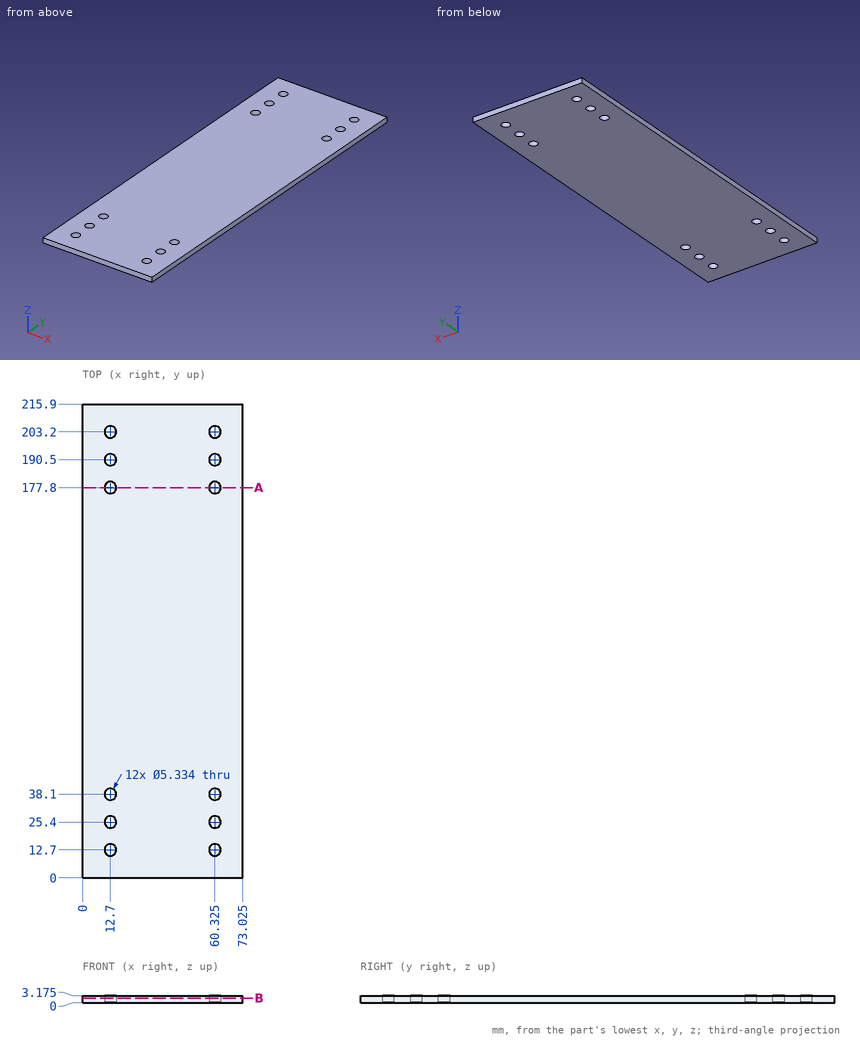
Part print with two shaded views. Sizes in mm from the minimum x, y, z corner. Coordinates: 2 decimals unless noted, no trailing zeros. Write each loop counter-clockwise with the first axis right and the second up, starting at its lowest first coordinate (ties: lowest second). Pieces come first, ordered by that corner, then holes.
1. Drill centre line: probe 1 along X at (y, z) = (177.8, 1.35) (3 decimals). Where is it in solid material? Low to high.
Answer block:
probe 1: x = 0 to 10.033, 15.367 to 57.658, 62.992 to 73.025
2. Drop a flat-ended pin along its axis: pin 1 (4.5 mm diameter, centred on x = 60.325, y = 25.4, fed in from +Z). Give the stop position or say it passes through.
Answer block:
pin 1: passes through
3. Band-saw the part on A-A, the plane y = 177.8. Give the cut face in (x, z) (3 decimals).
Answer block:
outline: (0, 0) - (10.033, 0) - (10.033, 3.175) - (0, 3.175) - close; (15.367, 0) - (57.658, 0) - (57.658, 3.175) - (15.367, 3.175) - close; (62.992, 0) - (73.025, 0) - (73.025, 3.175) - (62.992, 3.175) - close
4. Band-saw the part on B-B, the plane z = 2.15. Give the number of separate pieces and of enclosed holes in the cut face, and give its area (3 significant figures).
Answer block:
separate pieces: 1
enclosed holes: 12
area: 15,500 mm2
